```python
from build123d import *

# Parameters (mm, degrees)
BOSS_EXTRUDE1_DEPTH = 9.525
CAVITY1_START       = -9.525
CAVITY1_DEPTH       = 9.525


# Read off the part's stored shape, not the designer's step: Cavity1
with BuildPart() as part:
    # Sketch1 → Boss-Extrude1 (new body)
    with BuildSketch(Plane.XY):
        Polygon((-114.3, 19.05), (-60.325, 19.05), (-60.325, -19.05), (-114.3, -19.05), (-121.190985561, -19.05), (-111.454402918, 0), (-121.190985561, 19.05), align=None)
    extrude(amount=-BOSS_EXTRUDE1_DEPTH)

    # Cavity1 outline → Cavity1 (cut)
    with BuildSketch(Plane.XY.offset(CAVITY1_START)):
        with BuildLine():
            Line((-111.125, 15.875), (-60.325, 15.875))
            Line((-60.325, 15.875), (-60.325, 19.05))
            Line((-60.325, 19.05), (-121.190985561, 19.05))
            Line((-121.190985561, 19.05), (-111.454402918, 0))
            Line((-111.454402918, 0), (-121.190985561, -19.05))
            Line((-121.190985561, -19.05), (-60.325, -19.05))
            Line((-60.325, -19.05), (-60.325, -15.875))
            Line((-60.325, -15.875), (-111.125, -15.875))
            ThreePointArc((-111.125, -15.875), (-114.137069471, -13.704023157), (-113.03, -10.16))
            ThreePointArc((-113.03, -10.16), (-107.95, 0), (-113.03, 10.16))
            ThreePointArc((-113.03, 10.16), (-114.137069471, 13.704023157), (-111.125, 15.875))
        make_face()
    extrude(amount=CAVITY1_DEPTH, mode=Mode.SUBTRACT)


solid = part.part
```
The listing builds one solid part. Answer for the finished solid, in the listing's coordinates (mm). Give positions to 0.01 mm unless a question says otherwise; leave off trailing zeros. Write each loop counter-clockwise with the first axis right and the second up, starting at its lowest first coordinate (ties: lowest second). Pieces come first, ordered by that corner, then holes. Notation, with made-up numbers: (82, 53.25) - (104, 53.25) arc R21 ccw to (104, 90.25) - close; hole circle Ø8 at (12.25, -22.75). An arc over 180 degrees is marked (long way). Use one line per item in the form item = value. Start each with the question number.
1) Find section B-B on z = -2.25. Determine the outline of the cut face in (x, y) (3 decimals).
2) Find section C-C on y = 4.5. Determine the outline of the cut face in (x, z) (3 decimals), plus the area to 3 significant figures.
3) The mould has two halves that part along Y. Classify faces 1 (the face through (-114.119, -13.757, -4.829)), 2 (the face through (-107.95, -0.16, -4.83)), 3 (the face through (-86, 15.875, -5)), 4 (the face through (-87, 0, 0)): pulls with the +Y half, pulls with the -Y half, needs draft (parallel to the pull), parting line crosses it, or undercut.
4) Find section A-A on x = -110.5. Determine the outline of the cut face in (y, z) (3 decimals).
5) Find section D-D on y = -8. Determine the outline of the cut face in (x, z) (3 decimals), plus the area to 3 significant figures.
6) Consider line 1 along Y through (x, z) = (-111.5, -8.5); line 2 along Y through (x, z) = (-112, -5.75); line 3 along X through (y, z) = (2.5, -8) (1 decimal). Determine where each line is inside the solid, lowest interval first. Write a range as from..to.
7) A flat-ended cylindrical pin translates along its axis: pin 1 Ø6 at (x, y) = (-98, 0) entering from +Z. Find the tip coordinate at first contact, or state that the pin passes through.
Geometry results:
q1.outline = (-113.03, -10.16) arc R3.175 ccw to (-111.125, -15.875) - (-60.325, -15.875) - (-60.325, 15.875) - (-111.125, 15.875) arc R3.175 ccw to (-113.03, 10.16) arc R12.7 cw to start
q2.outline = (-108.774, -9.525) - (-60.325, -9.525) - (-60.325, 0) - (-108.774, 0) - close
q2.area = 461 mm2
q3.face_1 = undercut
q3.face_2 = undercut
q3.face_3 = pulls with the +Y half
q3.face_4 = needs draft
q4.outline = (-15.875, -9.525) - (-7.633, -9.525) - (-7.633, 0) - (-15.875, 0) - close; (7.633, -9.525) - (15.875, -9.525) - (15.875, 0) - (7.633, 0) - close
q5.outline = (-110.786, -9.525) - (-60.325, -9.525) - (-60.325, 0) - (-110.786, 0) - close
q5.area = 481 mm2
q6.line_1 = -15.85..-8.81, 8.81..15.85
q6.line_2 = -15.75..-9.3, 9.3..15.75
q6.line_3 = -108.2..-60.3
q7.pin_1 = 0
